Autodesk Inventor part; units mm, degrees
ref_plane "YZ Plane" through (0, 0, 0) normal (1, 0, 0) x (0, 1, 0)
ref_plane "XZ Plane" through (0, 0, 0) normal (0, 1, 0) x (-1, 0, 0)
ref_plane "XY Plane" through (0, 0, 0) normal (0, 0, 1) x (1, 0, 0)
sketch "Sketch1" plane through (0, 0, 0) normal (0, 1, 0) x (-1, 0, 0)
  line L0 (2.286, 0) -> (10.414, 0)
  line L1 (12.7, -2.286) -> (12.7, -10.414)
  line L2 (10.414, -12.7) -> (2.286, -12.7)
  line L3 (0, -10.414) -> (0, -2.286)
  line L4 (8.1534, -4.0386) -> (4.5466, -4.0386)
  line L5 (4.0386, -4.5466) -> (4.0386, -8.1534)
  line L6 (4.5466, -8.6614) -> (8.1534, -8.6614)
  line L7 (8.6614, -8.1534) -> (8.6614, -4.5466)
  line L8 (10.414, 0) -> (12.7, -2.286)
  line L9 (12.7, -10.414) -> (10.414, -12.7)
  line L10 (2.286, -12.7) -> (0, -10.414)
  line L11 (2.286, 0) -> (0, -2.286)
  arc A0 (8.6614, -4.5466) -> (8.1534, -4.0386) centre (8.1534, -4.5466) ccw
  arc A1 (8.1534, -8.6614) -> (8.6614, -8.1534) centre (8.1534, -8.1534) ccw
  arc A2 (4.0386, -8.1534) -> (4.5466, -8.6614) centre (4.5466, -8.1534) ccw
  arc A3 (4.5466, -4.0386) -> (4.0386, -4.5466) centre (4.5466, -4.5466) ccw
  line L12 (8.1534, -4.5466) -> (4.5466, -8.1534) construction
  line L13 (12.7, -10.414) -> (0, -2.286) construction
  point P0 (0, 0)
  point P1 (12.7, -12.7)
  point P2 (12.7, 0)
  point P3 (0, -12.7)
  point P4 (4.0386, -8.6614)
  point P5 (8.6614, -8.6614)
  point P6 (6.35, -6.35)
  dimension "d1" = 12.7
  dimension "d2" = 4.6228
  dimension "d3" = 2.286
  dimension "d4" = 2.286
  dimension "d5" = 2.286
  dimension "d6" = 2.286
  dimension "d7" = 2.286
  dimension "d8" = 2.286
  dimension "d9" = 2.286
  dimension "d10" = 2.286
  dimension "d11" = 0.508
extrude "Body" add sketch "Sketch1" along normal blind 1.5875
sketch "Sketch2" plane through (0, 1.5875, 0) normal (0, 1, 0) x (1, 0, 0)
  arc A0 (-8.1534, 8.6614) -> (-8.6614, 8.1534) centre (-8.1534, 8.1534) ccw construction
  arc A1 (-4.5466, 4.0386) -> (-4.0386, 4.5466) centre (-4.5466, 4.5466) ccw construction
  circle A2 centre (-6.35, 6.35) radius 2.1844
  line L0 (-8.1534, 8.1534) -> (-4.5466, 4.5466) construction
  point P0 (0, 0)
  dimension "d14" = 4.3688
surface extrude "Circle" sketch "Sketch2" against normal up to surface (1.5875 mm away) shown yes curves A2
pattern_linear "Rectangular Pattern1" count 2 spacing 12.7 along (0, 0, -1) of "Body", "Circle"
equation "\"d22\" = d19"
Here's how the part is built. I have some questions about the finished solid (model axes, mm). A direction names the side the tool comes from. Round coordinates to 2 decimals unless told otherwise and drop trailing zeros. Loops run counter-clockwise (first coordinate to the right, second up) from the corner with the lowest first, then second, coordinate; pieces in that order, holes last.
1. If we section it at C-C on y = 0.5: Count the separate pieces of the cut face and the enclosed holes in it, plus the area to 3 significant figures.
Answer list:
separate pieces: 1
enclosed holes: 2
area: 259 mm2
2. If I drill on line 1 along Z through (x, y) = (-7.5, 0.1); line 2 along X through (y, z) = (1.2, -18.5); line 3 along Z through (x, y) = (-12, 1.45), over which ranges is the centre line in solid material (lowest first)?
Answer list:
line 1: z = -25.4 to -21.36, -16.74 to -8.66, -4.04 to 0
line 2: x = -12.7 to -8.66, -4.04 to 0
line 3: z = -23.81 to -14.29, -11.11 to -1.59
3. We'd pull the mould along X, two halves only. Please class faces 1 (the face through (-1.159, 0.783, -13.827)), 2 (the face through (-8.661, 1, -6)), 3 (the face through (-12.7, 1, -6)): +X half, -X half, draft (parallel to the pull), parting line (faces both ways), or undercut.
Answer list:
face 1: +X half
face 2: undercut
face 3: -X half
4. Which directions (+Z, -Z, +X, -X, +Y, -Y) give clear straight access to the entire face, cutting with the end or side of a thin tool? Please do faces 4 (the face through (-1.159, 0.783, -11.573)), 5 (the face through (-6, 1, -8.661)), 6 (the face through (-11.541, 0.783, -13.827)), 7 (the face through (-12.7, 1, -19)).
Answer list:
face 4: +X, +Y, -Y
face 5: +Y, -Y
face 6: -X, +Y, -Y
face 7: +Z, -Z, -X, +Y, -Y
5. If we section it at D-D on z = -2: Write out the boundary of the cut face in (x, y), plus the area to 3 significant figures.
Answer list:
outline: (-12.41, 0) - (-0.29, 0) - (-0.29, 1.59) - (-12.41, 1.59) - close
area: 19.3 mm2
6. If we section it at A-A on z = -19.5: Write out the boundary of the cut face in (x, y).
Answer list:
outline: (-12.7, 0) - (-8.66, 0) - (-8.66, 1.59) - (-12.7, 1.59) - close; (-4.04, 0) - (0, 0) - (0, 1.59) - (-4.04, 1.59) - close
7. If we section it at B-B on x = -7.5: Write out the boundary of the cut face in (y, z), plus the area to 3 significant figures.
Answer list:
outline: (0, -25.4) - (1.59, -25.4) - (1.59, -21.36) - (0, -21.36) - close; (0, -16.74) - (1.59, -16.74) - (1.59, -8.66) - (0, -8.66) - close; (0, -4.04) - (1.59, -4.04) - (1.59, 0) - (0, 0) - close
area: 25.6 mm2
